from build123d import *

# Parameters (mm, degrees)
SKETCH1_W                 = 60
SKETCH1_H                 = 80
SKETCH1_R                 = 11
SKETCH1_R_2               = 1.5
BOSS_EXTRUDE1_DEPTH       = 10
M4X0_7_TAPPED_HOLE1_D     = 3.3
M4X0_7_TAPPED_HOLE1_DEPTH = 10.1
M4X0_7_TAPPED_HOLE1_TIP   = 0.991420021
CHAMFER1_SIZE             = 2


with BuildPart() as part:
    # Sketch1 → Boss-Extrude1 (new body)
    with BuildSketch(Plane.XY):
        with Locations((30, 40)):
            Rectangle(SKETCH1_W, SKETCH1_H)
        with Locations((30, 60)):
            Circle(SKETCH1_R, mode=Mode.SUBTRACT)
        with Locations((15, 75)):
            Circle(SKETCH1_R_2, mode=Mode.SUBTRACT)
        with Locations((45, 75)):
            Circle(SKETCH1_R_2, mode=Mode.SUBTRACT)
        with Locations((45, 45)):
            Circle(SKETCH1_R_2, mode=Mode.SUBTRACT)
        with Locations((15, 45)):
            Circle(SKETCH1_R_2, mode=Mode.SUBTRACT)
    extrude(amount=BOSS_EXTRUDE1_DEPTH)

    # M4x0.7 Tapped Hole1
    with Locations(Plane(origin=(0, 0, 0), x_dir=(-1, 0, 0), z_dir=(0, -1, 0))):
        with Locations((-8, -5), (-30, -5), (-52, -5)):
            Hole(M4X0_7_TAPPED_HOLE1_D / 2, depth=M4X0_7_TAPPED_HOLE1_DEPTH)
            with Locations((0, 0, -(M4X0_7_TAPPED_HOLE1_DEPTH + M4X0_7_TAPPED_HOLE1_TIP / 2))):  # 118° drill point
                Cone(0, M4X0_7_TAPPED_HOLE1_D / 2, M4X0_7_TAPPED_HOLE1_TIP, mode=Mode.SUBTRACT)

    # Chamfer1
    chamfer1_edges = [part.edges().sort_by_distance(p)[0] for p in [
        (13.5, 75, 10),
        (43.5, 75, 10),
        (43.5, 45, 10),
        (13.5, 45, 10),
    ]]
    chamfer(chamfer1_edges, length=CHAMFER1_SIZE)


solid = part.part
Work out the finished part from the listing and answer in its coordinate system (mm). A direction names the side the tool comes from. Coordinates: 2 decimals unless noted, no trailing zeros. Order: outer loops, then holes, each group sorted by start corner. A loop starts at its lowest first (then second) coordinate and runs counter-clockwise, first axis right, second up. Notation, with made-up numbers: (-8.75, 84) - (8.25, 84) arc R25 cw to (8.25, 117) - close; hole circle Ø3 at (22.5, 84). An arc over 180 degrees is marked (long way). Put each result on its own line as item: value. Start each with the question number.
1) Find section A-A (y = 60). Give the vertices of the cut face in (x, z), plus the area to 3 significant figures.
2) Find section D-D (x = 34.5). Give the vertices of the cut face in (y, z).
3) Find the intervals of material crossed by line 1 (X direction, y = 4, z = 5); line 2 (Y direction, x = 15, z = 6.5); line 3 (Y direction, x = 13.5, z = 9.5), in increasing order. Write a range as from..to.
4) Flat-ended cylindrical pins translate along their axes: pin 1 (10 mm diameter, centred on x = 25.5, y = 50.5, fed in from +Z); pin 2 (3.5 mm diameter, centred on x = 45, y = 45, fed in from +Z); pin 3 (4 mm diameter, centred on x = 15, y = 75, fed in from +Z). Find the tip coordinate at first contact, or state that the pin passes through.
5) For faces 4 (the cylindrical face through (6.69, 5.12, 6)), 5 (the flat face through (30, 41, 0)), determine the directions among +Z, -Z, +X, -X, +Y, -Y from which every point of the face is accessible in a straight line to the end or side of a thin tool.
6) Find section B-B (x = 15). Give the vertices of the cut face in (y, z).
7) For a pull along Z with two mould halves and no side action, classify faces 1 (the cylindrical face through (28.568, 70.906, 4.93)), 2 (the flat face through (30, 41, 10)), 3 (the conical face through (7.7, 10.9, 4.9)) as released by +Z, released by -Z, zero draft, split by the parting line, or undercut.
8) Find section C-C (y = 45). Give the vertices of the cut face in (x, z), plus the area to 3 significant figures.
Results list:
1. outline: (0, 0) - (19, 0) - (19, 10) - (0, 10) - close; (41, 0) - (60, 0) - (60, 10) - (41, 10) - close
1. area: 380 mm^2
2. outline: (0, 0) - (49.96, 0) - (49.96, 10) - (0, 10) - close; (70.04, 0) - (80, 0) - (80, 10) - (70.04, 10) - close
3. line 1: x = 0..6.35, 9.65..28.35, 31.65..50.35, 53.65..60
3. line 2: y = 0..43.5, 46.5..73.5, 76.5..80
3. line 3: y = 0..42.4, 47.6..72.4, 77.6..80
4. pin 1: stops at z = 10
4. pin 2: stops at z = 8.25
4. pin 3: stops at z = 8.5
5. face 4: -Y
5. face 5: -Z, +X, -X, +Y, -Y
6. outline: (0, 0) - (43.5, 0) - (43.5, 8) - (41.5, 10) - (0, 10) - close; (46.5, 0) - (73.5, 0) - (73.5, 8) - (71.5, 10) - (48.5, 10) - (46.5, 8) - close; (76.5, 0) - (80, 0) - (80, 10) - (78.5, 10) - (76.5, 8) - close
7. face 1: zero draft
7. face 2: released by +Z
7. face 3: undercut
8. outline: (0, 0) - (13.5, 0) - (13.5, 8) - (11.5, 10) - (0, 10) - close; (16.5, 0) - (43.5, 0) - (43.5, 8) - (41.5, 10) - (18.5, 10) - (16.5, 8) - close; (46.5, 0) - (60, 0) - (60, 10) - (48.5, 10) - (46.5, 8) - close
8. area: 532 mm^2
